The model under review builds one solid part; all positions refer to its coordinate system, in mm. A direction names the side the tool comes from. Round coordinates to 2 decimals unless told otherwise and drop trailing zeros. Order: outer loops, then holes, each group sorted by start corner. A loop starts at its lowest first (then second) coordinate and runs counter-clockwise, first axis right, second up. Notation, with made-up numbers: (14.5, -26) -> (68.5, -26) arc R24 ccw to (68.5, -16) -> close; hole circle Ø4 at (-10, -14). An arc over 180 degrees is marked (long way). Return JSON: item names as keys, results as strings. Group by question number.
from build123d import *

# Parameters (mm, degrees)
SKETCH1_W                       = 140
SKETCH1_H                       = 200
BOSS_EXTRUDE1_DEPTH             = 2
SKETCH4_R                       = 20
CUT_EXTRUDE1_DEPTH              = 1
CUT_EXTRUDE2_REACH              = 4
SKETCH6_R                       = 2
SKETCH2_W                       = 4.004504799
SKETCH2_H                       = 7.007808652
CUT_EXTRUDE4_DEPTH              = 1
CUT_EXTRUDE4_DEPTH_BACK         = 3
CUT_EXTRUDE5_DEPTH              = 2
SKETCH8_W                       = 10
SKETCH8_H                       = 10
SKETCH8_R                       = 1.5
BOSS_EXTRUDE2_DEPTH             = 4
BOSS_EXTRUDE4_DEPTH             = 5
BOSS_EXTRUDE5_DEPTH             = 23
CUT_EXTRUDE6_DEPTH              = 10
F_3_0MM_CLEARANCE_DOWEL_HOLE1_D = 3
CUT_EXTRUDE7_DEPTH              = 26
SKETCH18_W                      = 140
SKETCH18_H                      = 27.200459883
CUT_EXTRUDE8_DEPTH              = 26
CUT_EXTRUDE9_DEPTH              = 32
SKETCH20_R                      = 1.5
BOSS_EXTRUDE7_DEPTH             = 10
LPATTERN1_COUNT                 = 3
LPATTERN1_PITCH                 = 75
CUT_EXTRUDE10_DEPTH             = 2


with BuildPart() as part:
    # Sketch1 → Boss-Extrude1 (new body)
    with BuildSketch(Plane(origin=(0, 0, 0), x_dir=(1, 0, 0), z_dir=(0, 1, 0))):
        Rectangle(SKETCH1_W, SKETCH1_H)
    extrude(amount=BOSS_EXTRUDE1_DEPTH)

    # Sketch4 → Cut-Extrude1 (cut)
    with BuildSketch(Plane.XZ):
        with Locations((-43.968804066, -69.910192249)):
            Circle(SKETCH4_R)
    extrude(amount=-CUT_EXTRUDE1_DEPTH, mode=Mode.SUBTRACT)

    # Sketch6 → Cut-Extrude2 (cut, up to next)
    with BuildSketch(Plane.XZ, mode=Mode.PRIVATE) as cut_extrude2_sk1:
        with Locations((-63.414240549, -50.464755767)):
            Circle(SKETCH6_R)
    cut_extrude2_tool1 = extrude(cut_extrude2_sk1.sketch, amount=-CUT_EXTRUDE2_REACH, mode=Mode.PRIVATE) & part.part
    add(cut_extrude2_tool1.solids().sort_by_distance((-63.414241, 0, -50.464756))[0], mode=Mode.SUBTRACT)
    # Sketch6 → Cut-Extrude2 (cut, up to next)
    with BuildSketch(Plane.XZ, mode=Mode.PRIVATE) as cut_extrude2_sk2:
        with Locations((-24.523367583, -89.355628732)):
            Circle(SKETCH6_R)
    cut_extrude2_tool2 = extrude(cut_extrude2_sk2.sketch, amount=-CUT_EXTRUDE2_REACH, mode=Mode.PRIVATE) & part.part
    add(cut_extrude2_tool2.solids().sort_by_distance((-24.523368, 0, -89.355629))[0], mode=Mode.SUBTRACT)

    # Sketch2 → Cut-Extrude4 (cut, two sides)
    with BuildSketch(Plane(origin=(0, 2, 0), x_dir=(1, 0, 0), z_dir=(0, 1, 0))) as cut_extrude4_sk:
        Polygon((-15.389965741, 53.410192249), (-11.889965741, 59.472370076), (-22.282270586, 65.472370076), (-25.782270586, 59.410192249), align=None)
        with BuildLine():
            Line((-62, 80.655444566), (-66, 80.655444566))
            Line((-66, 80.655444566), (-66, 75.655444566))
            Line((-66, 75.655444566), (-63.125841306, 75.655444566))
            ThreePointArc((-63.125841306, 75.655444566), (-62.619676759, 77.131338127), (-62, 78.563282633))
            Line((-62, 78.563282633), (-62, 80.655444566))
        make_face()
        with Locations((21.429491924, 36.193920339)):
            Rectangle(SKETCH2_W, SKETCH2_H)
    extrude(amount=CUT_EXTRUDE4_DEPTH, mode=Mode.SUBTRACT)
    extrude(cut_extrude4_sk.sketch, amount=-CUT_EXTRUDE4_DEPTH_BACK, mode=Mode.SUBTRACT)

    # Sketch7 → Cut-Extrude5 (cut)
    with BuildSketch(Plane(origin=(0, 2, 0), x_dir=(1, 0, 0), z_dir=(0, 1, 0))):
        Polygon((-11.836174724, -52.702068722), (-14.572335871, -45.184527756), (23.015368961, -31.503722023), (25.751530107, -39.021262989), align=None)
        Polygon((-14.914356014, -44.244835135), (22.673348817, -30.564029402), (23.015368961, -31.503722023), (-14.572335871, -45.184527756), align=None)
    extrude(amount=-CUT_EXTRUDE5_DEPTH, mode=Mode.SUBTRACT)

    # Sketch8 → Boss-Extrude2 (add)
    with BuildSketch(Plane(origin=(10.197981142, 0, -3.711761585), x_dir=(0.342020143, 0, 0.939692621), z_dir=(-0.939692621, 0, 0.342020143))):
        with Locations((33.475534903, -5)):
            Rectangle(SKETCH8_W, SKETCH8_H)
        with Locations((33.475534903, -5)):
            Circle(SKETCH8_R, mode=Mode.SUBTRACT)
    boss_extrude2 = extrude(amount=-BOSS_EXTRUDE2_DEPTH)

    # Mirror1: Boss-Extrude2 across plane
    add(boss_extrude2.mirror(Plane(origin=(-8.595871274, 0, 3.128641281), x_dir=(0.342020143, 0, 0.939692621), z_dir=(-0.939692621, 0, 0.342020143))))

    # Sketch9 → Boss-Extrude4 (add)
    with BuildSketch(Plane(origin=(0, 0, 0), x_dir=(-1, 0, 0), z_dir=(0, -1, 0))):
        with BuildLine():
            Line((18.286185593, -17.803458652), (12.129823014, -34.717925827))
            ThreePointArc((12.129823014, -34.717925827), (8.284684721, -36.510943259), (6.491667289, -32.665804967))
            Line((6.491667289, -32.665804967), (12.648029869, -15.751337793))
            ThreePointArc((12.648029869, -15.751337793), (16.493168161, -13.95832036), (18.286185593, -17.803458652))
        make_face()
        with BuildLine():
            Line((16.406800352, -17.119418366), (10.250437772, -34.03388554))
            ThreePointArc((10.250437772, -34.03388554), (8.968725008, -34.631558017), (8.37105253, -33.349845253))
            Line((8.37105253, -33.349845253), (14.52741511, -16.435378079))
            ThreePointArc((14.52741511, -16.435378079), (15.809127874, -15.837705602), (16.406800352, -17.119418366))
        make_face(mode=Mode.SUBTRACT)
    boss_extrude4 = extrude(amount=BOSS_EXTRUDE4_DEPTH)

    # Mirror2: Boss-Extrude4 across plane
    add(boss_extrude4.mirror(Plane(origin=(-8.595871274, 0, 3.128641281), x_dir=(0.342020143, 0, 0.939692621), z_dir=(-0.939692621, 0, 0.342020143))))

    # Sketch10 → Boss-Extrude5 (add)
    with BuildSketch(Plane.XZ):
        Polygon((-28.465283288, -55.763077932), (-19.80502925, -50.763077932), (-23.80502925, -43.834874702), (-32.465283288, -48.834874702), align=None)
    boss_extrude5 = extrude(amount=BOSS_EXTRUDE5_DEPTH)

    # Sketch11 → Cut-Extrude6 (cut)
    with BuildSketch(Plane(origin=(-45.495083508, 0, -26.26659871), x_dir=(-0.5, 0, 0.866025404), z_dir=(-0.866025404, 0, -0.5))):
        with BuildLine():
            Line((-30.059600438, -20.004300783), (-30.059600438, -16.004300783))
            ThreePointArc((-30.059600438, -16.004300783), (-29.059600438, -15.004300783), (-28.059600438, -16.004300783))
            Line((-28.059600438, -16.004300783), (-28.059600438, -20.004300783))
            ThreePointArc((-28.059600438, -20.004300783), (-29.059600438, -21.004300783), (-30.059600438, -20.004300783))
        make_face()
        with BuildLine():
            Line((-30.059600438, -6.504300783), (-30.059600438, -2.504300783))
            ThreePointArc((-30.059600438, -2.504300783), (-29.059600438, -1.504300783), (-28.059600438, -2.504300783))
            Line((-28.059600438, -2.504300783), (-28.059600438, -6.504300783))
            ThreePointArc((-28.059600438, -6.504300783), (-29.059600438, -7.504300783), (-30.059600438, -6.504300783))
        make_face()
    cut_extrude6 = extrude(amount=-CUT_EXTRUDE6_DEPTH, mode=Mode.SUBTRACT)

    # Mirror3: Boss-Extrude5, Cut-Extrude6 across plane
    add(boss_extrude5.mirror(Plane(origin=(21.029800219, 0, -36.424682453), x_dir=(0.866025404, 0, 0.5), z_dir=(-0.5, 0, 0.866025404))))
    add(cut_extrude6.mirror(Plane(origin=(21.029800219, 0, -36.424682453), x_dir=(0.866025404, 0, 0.5), z_dir=(-0.5, 0, 0.866025404))), mode=Mode.SUBTRACT)

    # Ø3.0mm Clearance Dowel Hole1 (through all)
    with Locations(Plane(origin=(-89.742029537, 2, 119.499715795), x_dir=(1, 0, 0), z_dir=(0, 1, 0))):
        with Locations((23.542258378, 99.781049413), (25.594379238, 52.014538143), (70.699625036, 68.431505023), (70.526889417, 116.882056579), (111.491838386, 131.259989766), (119.586439667, 85.314281565), (155.294759257, 98.311047011), (152.806439447, 156.481766603), (65.878236217, 157.017664987), (102.576966028, 185.481766603), (52.347492608, 214.481766603), (25.242029537, 178.499715795)):
            Hole(F_3_0MM_CLEARANCE_DOWEL_HOLE1_D / 2)

    # Sketch16 → Cut-Extrude7 (cut, through all)
    with BuildSketch(Plane(origin=(0, 2, 0), x_dir=(1, 0, 0), z_dir=(0, 1, 0))):
        Polygon((-43.621778265, 110.124355653), (83.026139699, 110.124355653), (83.026139699, 36.903214828), (77, 40.483339502), align=None)
    extrude(amount=-CUT_EXTRUDE7_DEPTH, mode=Mode.SUBTRACT)

    # Sketch18 → Cut-Extrude8 (cut, through all)
    with BuildSketch(Plane(origin=(0, 2, 0), x_dir=(1, 0, 0), z_dir=(0, 1, 0))):
        with Locations((0, -86.399770058)):
            Rectangle(SKETCH18_W, SKETCH18_H)
    extrude(amount=-CUT_EXTRUDE8_DEPTH, mode=Mode.SUBTRACT)

    # Sketch19 → Cut-Extrude9 (cut, through all)
    with BuildSketch(Plane(origin=(-89.742029537, 8, 119.499715795), x_dir=(1, 0, 0), z_dir=(0, 1, 0))):
        with BuildLine():
            Line((44.742029537, 154.499715795), (44.742029537, 124.499715795))
            ThreePointArc((44.742029537, 124.499715795), (39.742029537, 119.499715795), (34.742029537, 124.499715795))
            Line((34.742029537, 124.499715795), (34.742029537, 154.499715795))
            ThreePointArc((34.742029537, 154.499715795), (39.742029537, 159.499715795), (44.742029537, 154.499715795))
        make_face()
    extrude(amount=-CUT_EXTRUDE9_DEPTH, mode=Mode.SUBTRACT)

    # Sketch20 → Boss-Extrude7 (add)
    with BuildSketch(Plane.ZY.offset(70)):
        with BuildLine():
            Line((55.358547654, -3), (55.358547654, 0))
            Line((55.358547654, 0), (62.358547654, 0))
            Line((62.358547654, 0), (62.358547654, -3))
            ThreePointArc((62.358547654, -3), (58.858547654, -6.5), (55.358547654, -3))
        make_face()
        with Locations((58.858547654, -3)):
            Circle(SKETCH20_R, mode=Mode.SUBTRACT)
    boss_extrude7 = extrude(amount=-BOSS_EXTRUDE7_DEPTH)

    # LPattern1: Boss-Extrude7 ×3
    with Locations(*[(0, 0, -i * LPATTERN1_PITCH) for i in range(1, LPATTERN1_COUNT)]):
        add(boss_extrude7)

    # Sketch22 → Cut-Extrude10 (cut)
    with BuildSketch(Plane(origin=(0, 2, 0), x_dir=(1, 0, 0), z_dir=(0, 1, 0))):
        Polygon((-14.914356014, -44.244835135), (-8.336507669, -41.850694132), (-16.544991108, -19.298071233), (-23.122839454, -21.692212236), align=None)
    extrude(amount=-CUT_EXTRUDE10_DEPTH, mode=Mode.SUBTRACT)


solid = part.part
Item 1: Wall thickness on line 1 along Y through (x, z) = (-4.5, -64.5); line 2 along Y through (x, z) = (-19.5, 41); line 3 along X through (y, z) = (-20.5, -51): over which ranges is each line inside the solid? List them lowest first.
Item 2: For faces 1 (the face through (-13.707, -1.505, -71.466)), 2 (the face through (6.951, 1.014, 36.286)), 3 (the face through (-14, 0, 28)), 4 (the face through (-12.07, -11.34, -74.01)), list the 3-axis set-ups (+Z, -Z, +X, -X, +Y, -Y) from which the entire face can be reached by the end or side of a thin tool; tool diameter is ignored.
Item 3: Consider section B-B on x = -50. State the section outline as (y, z) points.
Item 4: Consider section A-A on y = -12.75. State the section outline as (x, z) points.
Item 5: Insertion check: pin 1 Ø8 at (y, z) = (-20, -72) entering from -X; pin 2 Ø6 at (x, z) = (6, 12) entering from -Y; pin 3 Ø10 at (x, z) = (-33.5, -42) entering from -Y; pin 4 Ø2.5 at (x, z) = (12.83, -65.98) entering from -Y. Each pin has a flat end and moves straight along its axis. Give the tip position at first contact, or say it passes through.
Item 6: The part is to be moulded in two halves that separate along Z. For faces 5 (the face through (22.63, 1.014, -71.874)), 6 (the face through (-16.083, -5.07, 46.799)), 7 (the face through (-16.431, -2.465, 13.936)), say which applies: +Z half, -Z half, draft (parallel to the pull), parting line (faces both ways), or undercut.
Values:
{
 "1": {"line 1": "0 to 2", "line 2": "-10 to 2", "line 3": "-28.48 to -20.22"},
 "2": {"face 1": "none", "face 2": "+Y, -Y", "face 3": "+Y", "face 4": "-Z, +X, -Y"},
 "3": {"outline": "(0, -100) -> (2, -100) -> (2, -40) -> (0, -40) -> (0, -50.84) -> (1, -50.84) -> (1, -88.98) -> (0, -88.98) -> close; (0, 0) -> (2, 0) -> (2, 72.8) -> (0, 72.8) -> close"},
 "4": {"outline": "(-32.47, -48.83) -> (-28.47, -55.76) -> (-19.81, -50.76) -> (-23.81, -43.83) -> close; (-20.47, -69.62) -> (-16.47, -76.55) -> (-7.81, -71.55) -> (-11.81, -64.62) -> close"},
 "5": {"pin 1": "x = -20.47", "pin 2": "y = -5", "pin 3": "y = 0", "pin 4": "through"},
 "6": {"face 5": "-Z half", "face 6": "+Z half", "face 7": "undercut"}
}
